Can you work these out from the model? Positions are in its coordinate system, mm. A direction names the side the tool comes from. Round coordinates to 2 decimals unless told otherwise and drop trailing zeros. Loops run counter-clockwise (first coordinate to the right, second up) from the corner with the lowest first, then second, coordinate; pieces in that order, holes last.
(1) Which directions (+Z, -Z, +X, -X, +Y, -Y) give clear straight access to the entire face, cutting with the end or side of a thin tool? Please do faces 1 (the face through (-60, 20, 30)), 2 (the face through (-38.63, 37.91, 54.93)), 3 (the face through (-38.63, 37.91, 4.93)).
(2) I want a section at C-C on x = -43. Write out the boundary of the cut face in (y, z).
(3) I want a section at A-A on y = 30. Write out the boundary of the cut face in (x, z), plus the area to 3 significant figures.
(4) Will these pins go through, and if not, where does the flat tip stop? pin 1 Ø6 at (x, z) = (-49, 24.5) entering from +Y; pin 2 Ø14 at (x, y) = (-30, 30) entering from -Z; pin 3 Ø6 at (x, z) = (-44, 33.5) entering from +Y.
(5) If I drill on line 1 along X through (y, z) = (32.5, 3); line 2 along Y through (x, z) = (-32, 5); line 3 along Y through (x, z) = (-25, 7), over which ranges is the centre line in solid material (lowest first)?
(6) I want a section at B-B on z = 14.5. Write out the boundary of the cut face in (x, y).
(7) Thinking about a two-plate mould opening in Y: for faces 4 (the face through (-44.79, 53.414, 29.58)), 5 (the face through (-30, 30, 10)), 6 (the face through (0, 20, 30)), 7 (the face through (-30, 30, 50)), which applies, released by +Y, released by -Y, zero draft, split by the parting line, or undercut?
from build123d import *

# Parameters (mm, degrees)
F0_R     = 11.7054565065
F1_DEPTH = 60
F2_START = 10
F2_DEPTH = 40


# Not quite as in the source:
# - a feature names something its author has since deleted; it is built from what else it names


with BuildPart() as f1:
    # F0 (on Top) → F1 (new body)
    with BuildSketch(Plane.XY):
        Polygon((-60, 40.0004889347), (-60, 0), (0, 0), (0, 40), (-29.9997844001, 66.457757576), align=None)
        with Locations((-29.9997844001, 30)):
            Circle(F0_R, mode=Mode.SUBTRACT)
    extrude(amount=F1_DEPTH)

    # F0 (on Top) → F2 (join)
    with BuildSketch(Plane.XY.offset(F2_START)):
        with Locations((-29.9997844001, 30)):
            Circle(F0_R)
    extrude(amount=F2_DEPTH)


solid = f1.part
Filled sheet:
1. face 1: +Z, -Z, -X, +Y, -Y
1. face 2: +Z
1. face 3: -Z
2. outline: (0, 0) - (54.99, 0) - (54.99, 60) - (0, 60) - close
3. outline: (-60, 0) - (-41.71, 0) - (-41.71, 10) - (-18.29, 10) - (-18.29, 0) - (0, 0) - (0, 60) - (-18.29, 60) - (-18.29, 50) - (-41.71, 50) - (-41.71, 60) - (-60, 60) - close
3. area: 3,130 mm2
4. pin 1: stops at y = 52.35
4. pin 2: stops at z = 10
4. pin 3: stops at y = 56.76
5. line 1: x = -60 to -41.44, -18.56 to 0
5. line 2: y = 0 to 18.47, 41.53 to 64.69
5. line 3: y = 0 to 19.42, 40.58 to 62.05
6. outline: (-60, 0) - (0, 0) - (0, 40) - (-30, 66.46) - (-60, 40) - close
7. face 4: released by +Y
7. face 5: undercut
7. face 6: zero draft
7. face 7: undercut
